Model file for the job. Use its own axes, mm. Face numbers are marked on the shaded views. A direction names the side the tool comes from. Round coordinates to 2 decimals unless told otherwise and drop trailing zeros. Order: outer loops, then holes, each group sorted by start corner. A loop starts at its lowest first (then second) coordinate and runs counter-clockwise, first axis right, second up. Notation, with made-up numbers: M -34,13 L 18,13 A10 cw 18,30 Z; hole C 20.5,80.5 d10. An arc over 180 degrees is marked long. Return JSON: item names as keys, results as strings. Group by question number.
Item 1: Pull direction X, two halves, no side cores. Call the marked faces 4, 5 and 6: pulls with the +X half, pulls with the -X half, needs draft (parallel to the pull), parting line crosses it, or undercut.
Item 2: Slice it at D-D on y = 1.5. Write the cut outline in (x, z) (3 decimals).
Item 3: Slice it at A-A on z = -6.35. Write the cut outline in (x, y) (3 decimals).
Item 4: Pin check, flat tips, straight feed: pin 1 Ø3 at (x, z) = (35.5, -1.5) entering from +Y; pin 2 Ø6.5 at (x, z) = (7.5, -6) entering from +Y; pin 3 Ø1.5 at (y, z) = (13, -3.5) entering from +X. Stop position of each tip, or through.
Item 5: Probe line 1 along X through (y, z) = (1.75, -6.35) (3 decimals); line 2 along Z through (x, y) = (6.35, 4.25) (3 decimals); line 3 along X through (y, z) = (2.25, -7.25). List the from-to ranges inside material, lowest first.
Item 6: Slice it at B-B on x = 25.4. Write the cut outline in (y, z) (3 decimals).
Item 7: Which spindle directions (+Z, -Z, +X, -X, +Y, -Y) get a long thin tool onto all of the face, cutting with end or side? Do the marked faces 1, 2 and 3. Say none if no direction does.
Item 8: Slice it at C-C on z = -11.5. Write the cut outline in (x, y) (3 decimals), then the cut area to 3 significant figures.
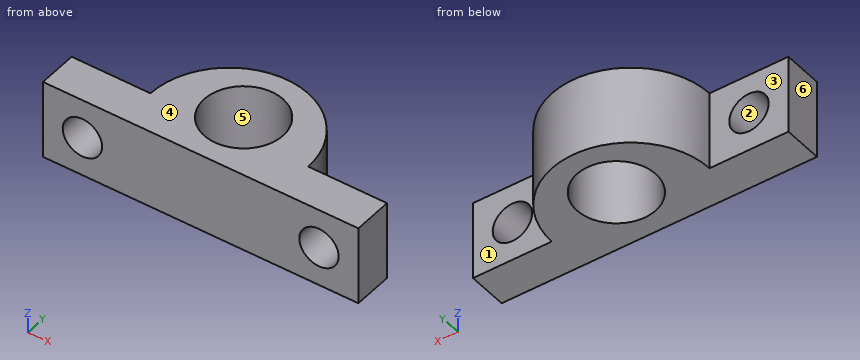
Autodesk Inventor part; units mm, degrees
ref_plane "YZ Plane" through (0, 0, 0) normal (1, 0, 0) x (0, 1, 0)
ref_plane "XZ Plane" through (0, 0, 0) normal (0, 1, 0) x (-1, 0, 0)
ref_plane "XY Plane" through (0, 0, 0) normal (0, 0, 1) x (1, 0, 0)
sketch "Sketch1" plane through (0, 0, 0) normal (0, 0, 1) x (1, 0, 0)
  line L0 (0, 0) -> (50.8, 0)
  line L1 (50.8, 0) -> (50.8, 6.35)
  line L2 (0, 6.35) -> (0, 0)
  arc A0 (38.1, 6.35) -> (12.7, 6.35) centre (25.4, 6.35) ccw
  line L3 (25.4, 6.35) -> (38.1, 6.35) construction
  line L4 (25.4, 6.35) -> (12.7, 6.35) construction
  line L5 (12.7, 6.35) -> (0, 6.35)
  line L6 (38.1, 6.35) -> (50.8, 6.35)
  circle A1 centre (25.4, 9.525) radius 6.35
  point P0 (25.4, 0)
  dimension "d0" = 50.8
  dimension "d2" = 12.7
  dimension "d3" = 180
  dimension "d4" = 6.35
  dimension "d5" = 12.7
  dimension "d6" = 9.525
extrude "Extrusion1" add sketch "Sketch1" against normal blind 12.7
sketch "Sketch2" plane through (0, 6.35, 0) normal (0, 1, 0) x (1, 0, 0)
  line L0 (0, 0) -> (0, 12.7)
  line L1 (50.8, 0) -> (50.8, 12.7)
  point P0 (6.35, 6.35)
  point P1 (44.45, 6.35)
  dimension "d9" = 6.35
  dimension "d10" = 6.35
hole "Hole1" at (6.35, 6.35, -6.35) at (44.45, 6.35, -6.35) direction (0, -1, 0) diameter 6.35 depth 25.4 tip angle 118
properties part number "axle bearing"
Output values:
{
 "1": {"face 4": "needs draft", "face 5": "undercut", "face 6": "pulls with the -X half"},
 "2": {"outline": "M 0,-12.7 L 50.8,-12.7 L 50.8,0 L 0,0 Z; hole C 6.35,-6.35 d6.35; hole C 44.45,-6.35 d6.35"},
 "3": {"outline": "M 0,0 L 3.175,0 L 3.175,6.35 L 0,6.35 Z; M 9.525,0 L 41.275,0 L 41.275,6.35 L 38.1,6.35 A12.7 ccw 12.7,6.35 L 9.525,6.35 Z; M 47.625,0 L 50.8,0 L 50.8,6.35 L 47.625,6.35 Z; hole C 25.4,9.525 d12.7"},
 "4": {"pin 1": "y = 15.7", "pin 2": "y = 6.35", "pin 3": "x = 36.65"},
 "5": {"line 1": "0 to 3.175, 9.525 to 41.275, 47.625 to 50.8", "line 2": "-12.7 to -9.525, -3.175 to 0", "line 3": "0 to 3.31, 9.39 to 41.41, 47.49 to 50.8"},
 "6": {"outline": "M 0,-12.7 L 3.175,-12.7 L 3.175,0 L 0,0 Z; M 15.875,-12.7 L 19.05,-12.7 L 19.05,0 L 15.875,0 Z"},
 "7": {"face 1": "+Z, -Z, +X, +Y", "face 2": "+Y, -Y", "face 3": "+Z, -Z, -X, +Y"},
 "8": {"outline": "M 0,0 L 50.8,0 L 50.8,6.35 L 38.1,6.35 A12.7 ccw 12.7,6.35 L 0,6.35 Z; hole C 25.4,9.525 d12.7", "area": "449 mm²"}
}
